from build123d import *

# Parameters (mm, degrees)
F0_W        = 367
F0_H        = 307
F0_W_2      = 340
F0_H_2      = 272
F1_DEPTH    = 25
F2_DEPTH    = 22
F3_R        = 2.4142135624
F4_W        = 339
F4_H        = 162.5
F5_DEPTH    = 31
F6_T1_DEPTH = 370.6623366275


# Not quite as in the source:
# - a fillet or chamfer that OpenCascade refuses, or shapes differently, is made with other operations: its cross-section is extruded or revolved along the edge and cut away or added


with BuildPart() as f1:
    # F0 (on Front) → F1 (new body)
    with BuildSketch(Plane.XZ):
        Rectangle(F0_W, F0_H)
        with Locations((0, 2)):
            Rectangle(F0_W_2, F0_H_2, mode=Mode.SUBTRACT)
    extrude(amount=F1_DEPTH)

    # F0 (on Front) → F2 (join)
    with BuildSketch(Plane.XZ):
        with Locations((0, 2)):
            Rectangle(F0_W_2, F0_H_2)
    extrude(amount=F2_DEPTH)

    # F3
    f3_edges = [f1.edges().sort_by_distance(p)[0] for p in [
        (-183.5, -25, 0),
        (183.5, -25, 0),
        (0, -25, 153.5),
        (0, -25, -153.5),
    ]]
    fillet(f3_edges, radius=F3_R)

    # F4 (on face) → F5 (join)
    with BuildSketch(Plane.XZ):
        with Locations((0, 7.95)):
            Rectangle(F4_W, F4_H)
    extrude(amount=-F5_DEPTH)

    # F6: fillet of radius 43.4558441227 on 2 edges, made by hand

    # F6_s2 → F6_t1 (cut)
    with BuildSketch(Plane.XY.offset(-177.3811683137)):
        with BuildLine():
            ThreePointArc((169.5, 0), (153.820674756, 22.3987797386), (127.8675326745, 31))
            Line((127.8675326745, 31), (169.5, 31))
            Line((169.5, 31), (169.5, 0))
        make_face()
        with BuildLine():
            ThreePointArc((-169.5, 0), (-153.820674756, 22.3987797386), (-127.8675326745, 31))
            Line((-127.8675326745, 31), (-169.5, 31))
            Line((-169.5, 31), (-169.5, 0))
        make_face()
    extrude(amount=F6_T1_DEPTH, mode=Mode.SUBTRACT)


solid = f1.part
Could you check a few things on this model? Use its own coordinates, in mm. A direction names the side the tool comes from. Give positions to 0.01 mm unless a question says otherwise; leave off trailing zeros. Order: outer loops, then holes, each group sorted by start corner. A loop starts at its lowest first (then second) coordinate and runs counter-clockwise, first axis right, second up.
1. Suppose I cut it at C-C (z = 121). List the corners of the cut face in (x, y) for me.
2. I need wall thicknesses on L1, parallel to Z at x = -78, y = 26.5; L2, parallel to Y at x = 11, z = -62; L3, parallel to Y at x = 42.5, z = 140. Which ranges of each line are inside material? Lowest first, please.
3. We'd pull the mould along X, two halves only. Please class faces 3 (the flat face through (-2, -22, 4)), 4 (the flat face through (-183.5, -11, -2)), 5 (the flat face through (-2, 15, -73.3)): pulls with the +X half, pulls with the -X half, needs draft (parallel to the pull), parting line crosses it, or undercut.
4. Suppose I cut it at B-B (x = -48.5). List the corners of the cut face in (y, z) for me.
5. Suppose I cut it at D-D (y = 23.5). List the corners of the cut face in (x, z) for me.
6. Suppose I cut it at A-A (z = 79.5). List the corners of the cut face in (x, y) for me.
7. Will these pins go through, and if not, where does the flat tip stop? P1, Ø2, axis at y = 14.5, z = -3.5, coming from the +X side; P2, Ø1.5, axis at x = -66.5, y = -23.5, coming from the +Z side; P3, Ø6, axis at y = 24, z = 45, coming from the -X side.
8. For faces 1 (the flat face through (-2, 15, 89.2)), 2 (the flat face through (183.5, -11, -2)), which set-ups out of +Z, -Z, +X, -X, +Y, -Y let a thin tool reach every point of the face, with its end or its side?
Solved:
1. outline: (-183.5, -22.59) arc R2.41 ccw to (-181.09, -25) - (-170, -25) - (-170, -22) - (170, -22) - (170, -25) - (181.09, -25) arc R2.41 ccw to (183.5, -22.59) - (183.5, 0) - (-183.5, 0) - close
2. L1: z = -73.3 to 89.2
2. L2: y = -22 to 31
2. L3: y = -25 to 0
3. face 3: undercut
3. face 4: pulls with the -X half
3. face 5: needs draft
4. outline: (-25, -151.09) arc R2.41 ccw to (-22.59, -153.5) - (0, -153.5) - (0, -73.3) - (31, -73.3) - (31, 89.2) - (0, 89.2) - (0, 153.5) - (-22.59, 153.5) arc R2.41 ccw to (-25, 151.09) - (-25, 138) - (-22, 138) - (-22, -134) - (-25, -134) - close
5. outline: (-152.27, -73.3) - (152.27, -73.3) - (152.27, 89.2) - (-152.27, 89.2) - close
6. outline: (-183.5, -22.59) arc R2.41 ccw to (-181.09, -25) - (-170, -25) - (-170, -22) - (170, -22) - (170, -25) - (181.09, -25) arc R2.41 ccw to (183.5, -22.59) - (183.5, 0) - (169.5, 0) arc R43.46 ccw to (127.87, 31) - (-127.87, 31) arc R43.46 ccw to (-169.5, 0) - (-183.5, 0) - close
7. P1: stops at x = 162.72
7. P2: stops at z = 153.49
7. P3: stops at x = -155.6
8. face 1: +Z, +X, -X, +Y
8. face 2: +Z, -Z, +X, +Y, -Y
